For this review, take the finished solid that the model builds, in its own axes (mm). Coordinates: 2 decimals unless noted, no trailing zeros. Write each loop counter-clockwise with the first axis right and the second up, starting at its lowest first coordinate (ties: lowest second). Pieces come first, ordered by that corner, then holes. Notation, with made-up numbers: (1, 25) -> (6, 25) arc R34 ccw to (6, 59) -> close; hole circle Ø10 at (9.25, 44.5). An arc over 180 degrees is marked (long way). Put each result on its own line as item: value. Start each with the question number.
Item 1: Consider section A-A on z = -21.59. Give the boundary of the cut face in (x, y) (3 decimals).
Item 2: Consider section D-D on z = -14.5. Give the boundary of the cut face in (x, y) (3 decimals).
Item 3: Consider section C-C on x = 26.67. Give the boundary of the cut face in (y, z) (3 decimals), and give its area (3 significant figures).
Item 4: Consider section B-B on y = 1.8. Give the boundary of the cut face in (x, z), and give its area (3 significant figures).
Item 5: To check wall thickness, follow L1, parallel to X at y = 0.9, z = -21.59; L2, parallel to X at y = 1.6, z = -36.5; L3, parallel to Z at x = 5, y = 2.3. State the ranges of each line that lie inside material, in increasing order.
Item 6: The part is to be moulded in two halves that separate along Z. For faces 1 (the cylindrical face through (34.874, 1.565, -5.816)), 2 (the cylindrical face through (0, 1.6, -21.5)), 3 (the cylindrical face through (26.41, 1.57, -43.18)), 4 (the cylindrical face through (4.79, 1.57, -23.82)), say which applies: +Z half, -Z half, draft (parallel to the pull), parting line (faces both ways), or undercut.
Item 7: Insertion check: P1, Ø12, axis at x = 43.5, z = -17, coming from the -Y side; P2, Ø3.5, axis at x = 5.08, z = -21.59, coming from the +Y side; P3, Ø1.5, axis at x = 10, y = 1, coming from the -Z side. Each pin has a flat end and moves straight along its axis. Give the tip position at first contact, or say it passes through.
```python
from build123d import *

# Parameters (mm, degrees)
SKETCH1_R           = 2.25
SKETCH1_R_2         = 17.78
BOSS_EXTRUDE1_DEPTH = 3.175


with BuildPart() as part:
    # Sketch1 → Boss-Extrude1 (new body)
    with BuildSketch(Plane(origin=(0, 0, 0), x_dir=(1, 0, 0), z_dir=(0, 1, 0))):
        with BuildLine():
            Line((52.144705882, 18.316552245), (43.18, 7.677847039))
            ThreePointArc((43.18, 7.677847039), (26.67, 0), (10.16, 7.677847039))
            Line((10.16, 7.677847039), (1.195294118, 18.316552245))
            ThreePointArc((1.195294118, 18.316552245), (0, 21.59), (1.195294118, 24.863447755))
            Line((1.195294118, 24.863447755), (10.16, 35.502152961))
            ThreePointArc((10.16, 35.502152961), (26.67, 43.18), (43.18, 35.502152961))
            Line((43.18, 35.502152961), (52.144705882, 24.863447755))
            ThreePointArc((52.144705882, 24.863447755), (53.34, 21.59), (52.144705882, 18.316552245))
        make_face()
        with Locations((48.26, 21.59)):
            Circle(SKETCH1_R, mode=Mode.SUBTRACT)
        with Locations((5.08, 21.59)):
            Circle(SKETCH1_R, mode=Mode.SUBTRACT)
        with Locations((26.67, 21.59)):
            Circle(SKETCH1_R_2, mode=Mode.SUBTRACT)
    extrude(amount=BOSS_EXTRUDE1_DEPTH)


solid = part.part
```
Return value:
1. outline: (0, 0) -> (2.83, 0) -> (2.83, 3.175) -> (0, 3.175) -> close; (7.33, 0) -> (8.89, 0) -> (8.89, 3.175) -> (7.33, 3.175) -> close; (44.45, 0) -> (46.01, 0) -> (46.01, 3.175) -> (44.45, 3.175) -> close; (50.51, 0) -> (53.34, 0) -> (53.34, 3.175) -> (50.51, 3.175) -> close
2. outline: (4.411, 0) -> (10.365, 0) -> (10.365, 3.175) -> (4.411, 3.175) -> close; (42.975, 0) -> (48.929, 0) -> (48.929, 3.175) -> (42.975, 3.175) -> close
3. outline: (0, -43.18) -> (3.175, -43.18) -> (3.175, -39.37) -> (0, -39.37) -> close; (0, -3.81) -> (3.175, -3.81) -> (3.175, 0) -> (0, 0) -> close
3. area: 24.2 mm^2
4. outline: (1.2, -24.86) -> (10.16, -35.5) arc R21.59 ccw to (43.18, -35.5) -> (52.14, -24.86) arc R5.08 ccw to (52.14, -18.32) -> (43.18, -7.68) arc R21.59 ccw to (10.16, -7.68) -> (1.2, -18.32) arc R5.08 ccw to start; hole circle Ø4.5 at (5.08, -21.59); hole circle Ø35.56 at (26.67, -21.59); hole circle Ø4.5 at (48.26, -21.59)
4. area: 565 mm^2
5. L1: 0 to 2.83, 7.33 to 8.89, 44.45 to 46.01, 50.51 to 53.34
5. L2: 11.06 to 16.98, 36.36 to 42.28
5. L3: -29.38 to -23.84, -19.34 to -13.8
6. face 1: undercut
6. face 2: parting line
6. face 3: -Z half
6. face 4: undercut
7. P1: y = 0
7. P2: through
7. P3: z = -36.17
